The drawing under review shows one solid part. Ordinate dimensions are in mm from its lowest x, y, z. A direction names the side the tool comes from. Coordinates: 2 decimals unless noted, no trailing zeros. Write each loop counter-clockwise with the first axis right and the second up, starting at its lowest first coordinate (ties: lowest second). Pieces come first, ordered by that corner, then holes.
1) Add section D-D, the plane x = 102.5. State the section outline as (y, z) points.
2) For line 1 (Z direction, x = 30, y = 93.5); line 2 (X direction, y = 58.5, z = 163.5); line 3 (Y direction, x = 60, z = 35), list the stretches that pass through material, from the lowest coordinate up.
3) Add section C-C, the plane z = 62. State the section outline as (x, y) points, then the cut area to 3 significant figures.
4) Add section A-A, the plane y = 65.5. State the section outline as (x, z) points.
5) For P1, Ø12, axis at x = 56, z = 30, coming from the -Y side; P2, Ø3, axis at y = 88.5, z = 31.5, coming from the -X side; P3, Ø12, axis at x = 88, z = 89.5, coming from the -Y side, all flat-tipped, find the tip position at first contact; note any pin that passes through.
6) Machinability: for the marked faces 1 and 2, which of the approach directions +Z, -Z, +X, -X, +Y, -Y give a long, thin tool a straight path to every point of the face, cutting with its end or side? Answer none if there is none.
7) Add section B-B, the plane x = 83. State the section outline as (y, z) points.
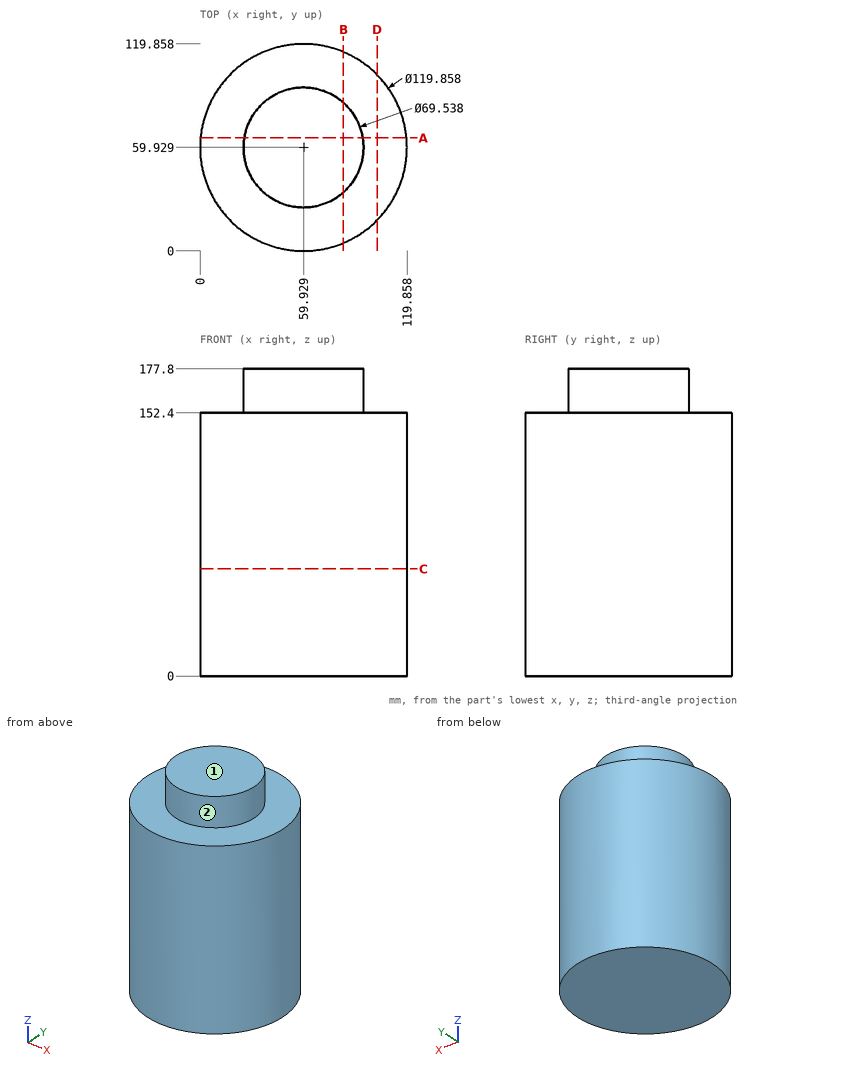
Geometry results:
1. outline: (17.75, 0) - (102.11, 0) - (102.11, 152.4) - (17.75, 152.4) - close
2. line 1: z = 0 to 152.4
2. line 2: x = 25.19 to 94.67
2. line 3: y = 0 to 119.86
3. outline: circle Ø119.86 at (59.93, 59.93)
3. area: 11,300 mm2
4. outline: (0.26, 0) - (119.6, 0) - (119.6, 152.4) - (94.25, 152.4) - (94.25, 177.8) - (25.61, 177.8) - (25.61, 152.4) - (0.26, 152.4) - close
5. P1: stops at y = 0
5. P2: stops at x = 6.46
5. P3: stops at y = 4.21
6. face 1: +Z, +X, -X, +Y, -Y
6. face 2: +Z
7. outline: (4.62, 0) - (115.24, 0) - (115.24, 152.4) - (85.94, 152.4) - (85.94, 177.8) - (33.92, 177.8) - (33.92, 152.4) - (4.62, 152.4) - close
